The drawing under review shows one solid part. Ordinate dimensions are in mm from its lowest x, y, z. A direction names the side the tool comes from. Give positions to 0.01 mm unless a question says otherwise; leave off trailing zeros. Order: outer loops, then holes, each group sorted by start corner. A loop starts at its lowest first (then second) coordinate and runs counter-clockwise, first axis right, second up. Notation, with made-up numbers: (43.25, -33) -> (65.25, -33) arc R25 cw to (65.25, -13) -> close; hole circle Ø3 at (-34.5, 32.5). An arc over 180 degrees is marked (long way). Return JSON: item names as keys, results as strings. Group by question number.
1) Add section B-B (z = 102). Give the boundary of the cut face in (x, y).
2) Insertion check: P1, Ø10, axis at y = 48, z = 77, coming from the +X side; P2, Ø3.5, axis at x = 11.5, z = 15, coming from the -Y side; P3, Ø1.5, axis at x = 5, y = 7.5, coming from the +Z side; P4, Ø9.5, axis at x = 20, y = 15, coming from the -Z side. Each pin has a flat end and moves straight along its axis. Give the tip position at first contact, or say it passes through.
3) Add section A-A (x = 20). Give the boundary of the cut face in (y, z).
4) Add section D-D (z = 76). Give the boundary of the cut face in (x, y).
5) To check wall thickness, follow line 1 along Z through (x, y) = (28, 56); line 2 along X through (y, z) = (56.6, 15); line 3 along X through (y, z) = (56, 102). State the ranges of each line that lie inside material, in increasing order.
6) Add section C-C (y = 34.5). Give the boundary of the cut face in (x, z), then the cut area to 3 significant figures.
7) For the marked faces 1 and 2, list the 3-axis set-ups (+Z, -Z, +X, -X, +Y, -Y) from which the entire face can be reached by the end or side of a thin tool; tool diameter is ignored.
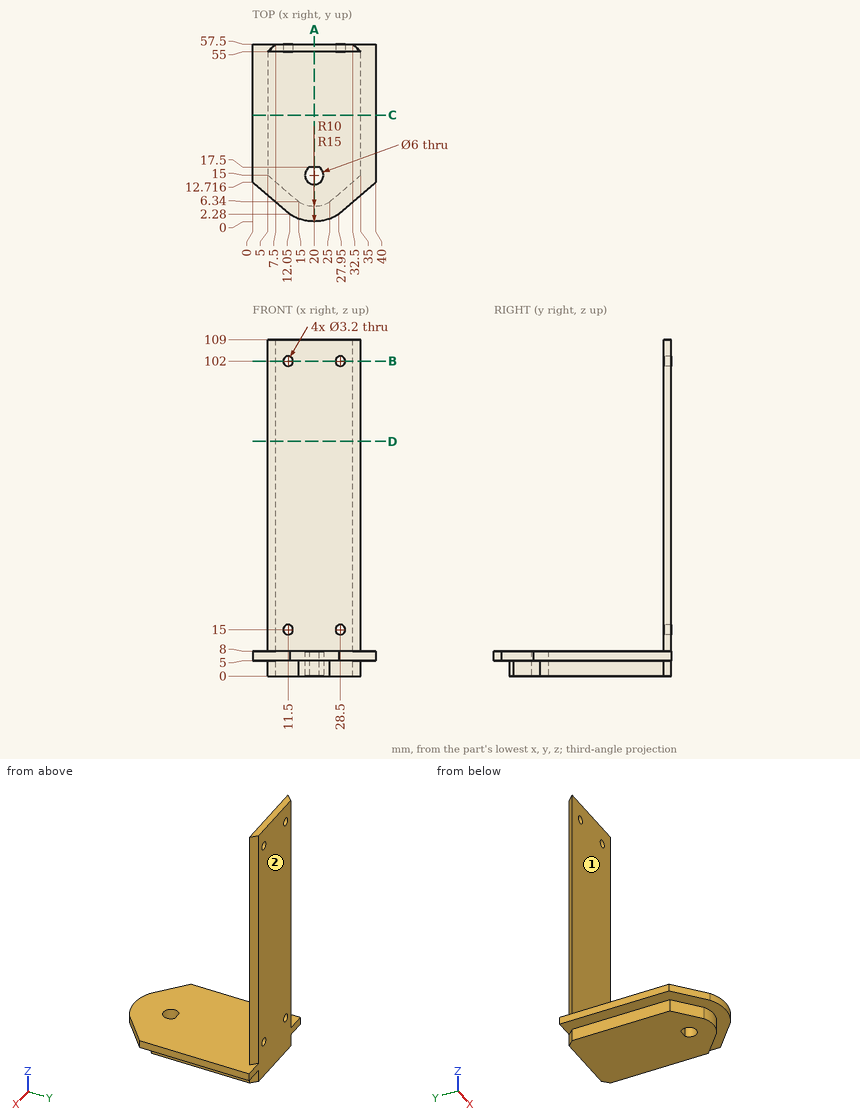
Evaluation:
{
 "1": {"outline": "(5, 55) -> (9.9, 55) -> (9.9, 57.5) -> (7.5, 57.5) -> close; (13.1, 55) -> (26.9, 55) -> (26.9, 57.5) -> (13.1, 57.5) -> close; (30.1, 55) -> (35, 55) -> (32.5, 57.5) -> (30.1, 57.5) -> close"},
 "2": {"P1": "through", "P2": "y = 55", "P3": "z = 8", "P4": "z = 0"},
 "3": {"outline": "(0, 5) -> (5, 5) -> (5, 0) -> (12, 0) -> (12, 8) -> (0, 8) -> close; (17.5, 0) -> (57.5, 0) -> (57.5, 109) -> (55, 109) -> (55, 8) -> (17.5, 8) -> close"},
 "4": {"outline": "(5, 55) -> (35, 55) -> (32.5, 57.5) -> (7.5, 57.5) -> close"},
 "5": {"line 1": "0 to 13.48, 16.52 to 100.48, 103.52 to 109", "line 2": "6.6 to 9.9, 13.1 to 26.9, 30.1 to 33.4", "line 3": "6 to 9.9, 13.1 to 26.9, 30.1 to 34"},
 "6": {"outline": "(0, 5) -> (5, 5) -> (5, 0) -> (35, 0) -> (35, 5) -> (40, 5) -> (40, 8) -> (0, 8) -> close", "area": "270 mm^2"},
 "7": {"face 1": "+Z, +X, -X, -Y", "face 2": "+Z, -Z, +X, -X, +Y"}
}
